```python
from build123d import *

# Parameters (mm, degrees)
SKETCH1_W           = 40
SKETCH1_H           = 35
BOSS_EXTRUDE1_DEPTH = 10
F_3DSKETCH1_R       = 2.25
CUT_EXTRUDE1_DEPTH  = 5
F_3DSKETCH2_R       = 5
CUT_EXTRUDE2_DEPTH  = 5


with BuildPart() as part:
    # Sketch1 → Boss-Extrude1 (new body)
    with BuildSketch(Plane(origin=(0, 0, 0), x_dir=(1, 0, 0), z_dir=(0, 1, 0))):
        Rectangle(SKETCH1_W, SKETCH1_H)
    extrude(amount=BOSS_EXTRUDE1_DEPTH)

    # 3DSketch1 → Cut-Extrude1 (cut)
    with BuildSketch(Plane(origin=(-7.5, 10, 0), x_dir=(1, 0, 0), z_dir=(0, -1, 0))):
        with Locations(Location((0, 0, 0), (0, 0, 90))):
            Circle(F_3DSKETCH1_R)
        with Locations(Location((15, 0, 0), (0, 0, 90))):
            Circle(F_3DSKETCH1_R)
    extrude(amount=CUT_EXTRUDE1_DEPTH, mode=Mode.SUBTRACT)

    # 3DSketch2 → Cut-Extrude2 (cut)
    with BuildSketch(Plane(origin=(-7.5, 0, 0), x_dir=(1, 0, 0), z_dir=(0, -1, 0))):
        with Locations(Location((0, 0, 0), (0, 0, 90))):
            Circle(F_3DSKETCH2_R)
        with Locations(Location((15, 0, 0), (0, 0, 90))):
            Circle(F_3DSKETCH2_R)
    extrude(amount=-CUT_EXTRUDE2_DEPTH, mode=Mode.SUBTRACT)


solid = part.part
```
Build history of the part. All positions in model axes, mm. A direction names the side the tool comes from. Round coordinates to 2 decimals unless told otherwise and drop trailing zeros. Loops run counter-clockwise (first coordinate to the right, second up) from the corner with the lowest first, then second, coordinate; pieces in that order, holes last.
Item 1: Two-plate mould, pull along Z, no slides. Class faces 3 (the face through (0, 5, 17.5)), 4 (the face through (-9.397, 7.535, 1.21)), 5 (the face through (0, 10, 0)): released by +Z, released by -Z, zero draft, split by the parting line, or undercut.
Item 2: Saw through at B-B (z = 0). List the corners of the cut face in (x, y).
Item 3: Pin check, flat tips, straight feed: P1, Ø11.5, axis at x = 7.5, z = 0, coming from the -Y side; P2, Ø5, axis at x = -9.5, z = 0.5, coming from the -Y side. Stop position of each tip, or through.
Item 4: Saw through at D-D (x = -7). List the corners of the cut face in (y, z).
Item 5: Saw through at A-A (x = 7.5). List the corners of the cut face in (y, z), then the cut area to 4 significant figures.
Item 6: Saw through at C-C (y = 1.75). List the corners of the cut face in (x, z).
Item 7: Which spindle directions (+Z, -Z, +X, -X, +Y, -Y) get a long thin tool onto all of the face, cutting with end or side? Do faces 1 (the face through (20, 5, 0)), 2 (the face through (-6, 5, 2)). Say none if no direction does.
Item 8: Drill centre lines: line 1 along X through (y, z) = (2, 0); line 2 along X through (y, z) = (7.45, 0); line 3 along Y through (x, z) = (12, 1). Where is each one in solid material? Low to high.
Worked answers:
1. face 3: released by +Z
1. face 4: undercut
1. face 5: zero draft
2. outline: (-20, 0) - (-12.5, 0) - (-12.5, 5) - (-9.75, 5) - (-9.75, 10) - (-20, 10) - close; (-5.25, 5) - (-2.5, 5) - (-2.5, 0) - (2.5, 0) - (2.5, 5) - (5.25, 5) - (5.25, 10) - (-5.25, 10) - close; (9.75, 5) - (12.5, 5) - (12.5, 0) - (20, 0) - (20, 10) - (9.75, 10) - close
3. P1: stops at y = 0
3. P2: stops at y = 5
4. outline: (0, -17.5) - (10, -17.5) - (10, -2.19) - (5, -2.19) - (5, -4.97) - (0, -4.97) - close; (0, 4.97) - (5, 4.97) - (5, 2.19) - (10, 2.19) - (10, 17.5) - (0, 17.5) - close
5. outline: (0, -17.5) - (10, -17.5) - (10, -2.25) - (5, -2.25) - (5, -5) - (0, -5) - close; (0, 5) - (5, 5) - (5, 2.25) - (10, 2.25) - (10, 17.5) - (0, 17.5) - close
5. area: 277.5 mm2
6. outline: (-20, -17.5) - (20, -17.5) - (20, 17.5) - (-20, 17.5) - close; hole circle Ø10 at (-7.5, 0); hole circle Ø10 at (7.5, 0)
7. face 1: +Z, -Z, +X, +Y, -Y
7. face 2: -Y
8. line 1: x = -20 to -12.5, -2.5 to 2.5, 12.5 to 20
8. line 2: x = -20 to -9.75, -5.25 to 5.25, 9.75 to 20
8. line 3: y = 5 to 10
